Here's how the part is built. I have some questions about the finished solid (model axes, mm). A direction names the side the tool comes from. Coordinates: 2 decimals unless noted, no trailing zeros. Write each loop counter-clockwise with the first axis right and the second up, starting at its lowest first coordinate (ties: lowest second). Pieces come first, ordered by that corner, then holes. Notation, with made-up numbers: (81.25, 15.5) -> (137.25, 15.5) arc R25 ccw to (137.25, 46.5) -> close; hole circle Ø5 at (30, 64). An arc over 180 degrees is marked (long way). Use a Markdown table: item, result. Add a question column.
Item 1: Imagine slicing it at D-D, the plane x = -17. Write out the boundary of the cut face in (y, z).
Item 2: On a 3-axis mill with a long thin cutter (end or side, diameter ignored), from which of +Z, -Z, +X, -X, +Y, -Y can I reach the whole of each face in a straight line? I mean faces 1 (the flat face through (0, 0, 11.43)), 2 (the flat face through (-34.265, 26.789, -0.196)), 3 (the flat face through (-18.446, -1, -3)). Say none if no direction works.
Item 3: If I drill on line 1 along Y through (x, z) = (0, 13.3); line 2 along Z through (x, y) = (-8, -6); line 3 along X through (y, z) = (5, 1.5), over which ranges is the centre line in solid material (lowest first)? Write a range as from..to.
Item 4: If we mould it in two halves opening along Y, with no side actions, what happens to faces 4 (the flat face through (0, 52.512, 0)), 5 (the flat face through (-10.725, -1, -3)), 6 (the flat face through (0, 19, 13.97))? For each: pulls with the +Y half, pulls with the -Y half, needs draft (parallel to the pull), parting line crosses it, or undercut.
Item 5: Imagine slicing it at B-B, the plane x = 0. Write out the boundary of the cut face in (y, z), and give its area (3 significant figures).
Item 6: Imagine slicing it at A-A, the plane z = 7. Write out the boundary of the cut face in (x, y), and give its area (3 significant figures).
Item 7: Imagine slicing it at C-C, the plane y = 0. Write out the boundary of the cut face in (x, z).
Item 8: Will these pins go through, and if not, where does the flat tip stop? pin 1 Ø5 at (x, z) = (5, -10.5) entering from -Y; pin 2 Ø10 at (y, z) = (23, -10.5) entering from -X; pin 3 Ø2 at (y, z) = (8, 10.5) entering from +X.
```python
from build123d import *

# Parameters (mm, degrees)
BOSS_EXTRUDE1_DEPTH      = 13.97
BOSS_EXTRUDE1_DEPTH_BACK = 13.97
SKETCH3_R                = 10.16
CUT_EXTRUDE1_DEPTH       = 2.54
SKETCH5_W                = 7.720577833
SKETCH5_H                = 11.69140021
CUT_EXTRUDE3_DEPTH       = 22.098


with BuildPart() as part:
    # Sketch2 → Boss-Extrude1 (new, two sides: drawn at the far end of the back side and taken through both)
    with BuildSketch(Plane.XY.offset(-BOSS_EXTRUDE1_DEPTH_BACK)):
        with BuildLine():
            Line((-35.51563317, 1.775781659), (-32.97880223, 52.512400474))
            Line((-32.97880223, 52.512400474), (32.97880223, 52.512400474))
            Line((32.97880223, 52.512400474), (35.51563317, 1.775781659))
            ThreePointArc((35.51563317, 1.775781659), (0, -35.56), (-35.51563317, 1.775781659))
        make_face()
    extrude(amount=BOSS_EXTRUDE1_DEPTH + BOSS_EXTRUDE1_DEPTH_BACK)

    # Sketch3 → Cut-Extrude1 (cut)
    with BuildSketch(Plane.XY.offset(13.97)):
        Circle(SKETCH3_R)
    extrude(amount=-CUT_EXTRUDE1_DEPTH, mode=Mode.SUBTRACT)

    # Sketch5 → Cut-Extrude3 (cut)
    with BuildSketch(Plane(origin=(0, 0, -13.97), x_dir=(-1, 0, 0), z_dir=(0, 0, -1))):
        with Locations((14.585332616, -1.114418504)):
            Rectangle(SKETCH5_W, SKETCH5_H)
    extrude(amount=-CUT_EXTRUDE3_DEPTH, mode=Mode.SUBTRACT)


solid = part.part
```
Ans:
| question | item | result |
|---|---|---|
| 1 | outline | (-31.23, -13.97) -> (-6.96, -13.97) -> (-6.96, 8.13) -> (4.73, 8.13) -> (4.73, -13.97) -> (52.51, -13.97) -> (52.51, 13.97) -> (-31.23, 13.97) -> close |
| 2 | face 1 | +Z |
| 2 | face 2 | +Z, -Z, -X, +Y |
| 2 | face 3 | -Z |
| 3 | line 1 | y = -35.56..-10.16, 10.16..52.51 |
| 3 | line 2 | z = -13.97..11.43 |
| 3 | line 3 | x = -35.35..35.35 |
| 4 | face 4 | pulls with the +Y half |
| 4 | face 5 | undercut |
| 4 | face 6 | needs draft |
| 5 | outline | (-35.56, -13.97) -> (52.51, -13.97) -> (52.51, 13.97) -> (10.16, 13.97) -> (10.16, 11.43) -> (-10.16, 11.43) -> (-10.16, 13.97) -> (-35.56, 13.97) -> close |
| 5 | area | 2,410 mm^2 |
| 6 | outline | (-35.52, 1.78) arc R35.56 ccw (long way) to (35.52, 1.78) -> (32.98, 52.51) -> (-32.98, 52.51) -> close; hole (-18.45, -6.96) -> (-10.73, -6.96) -> (-10.73, 4.73) -> (-18.45, 4.73) -> close |
| 6 | area | 5,500 mm^2 |
| 7 | outline | (-35.56, -13.97) -> (-18.45, -13.97) -> (-18.45, 8.13) -> (-10.73, 8.13) -> (-10.73, -13.97) -> (35.56, -13.97) -> (35.56, 13.97) -> (10.16, 13.97) -> (10.16, 11.43) -> (-10.16, 11.43) -> (-10.16, 13.97) -> (-35.56, 13.97) -> close |
| 8 | pin 1 | stops at y = -35.47 |
| 8 | pin 2 | stops at x = -34.7 |
| 8 | pin 3 | stops at x = 35.25 |
